```python
from build123d import *

# Parameters (mm, degrees)
SKETCH1_R           = 9
SKETCH1_R_2         = 6
BOSS_EXTRUDE1_DEPTH = 30


with BuildPart() as part:
    # Sketch1 → Boss-Extrude1 (new body)
    # profile 1 of 3: a face of its own
    with BuildSketch(Plane.XY):
        Circle(SKETCH1_R)
        Circle(SKETCH1_R_2, mode=Mode.SUBTRACT)
    # profile 2 of 3: a face of its own
    with BuildSketch(Plane.XY):
        with BuildLine():
            Line((-3.31662479, -5), (-3.31662479, 5))
            ThreePointArc((-3.31662479, 5), (-6, 0), (-3.31662479, -5))
        make_face()
    # profile 3 of 3: a face of its own
    with BuildSketch(Plane.XY):
        with BuildLine():
            ThreePointArc((6, 0), (5.286764074, 2.837274331), (3.31662479, 5))
            Line((3.31662479, 5), (3.31662479, -5))
            ThreePointArc((3.31662479, -5), (5.286764074, -2.837274331), (6, 0))
        make_face()
    extrude(amount=BOSS_EXTRUDE1_DEPTH)


solid = part.part
```
Geometry: final body of the model. Coordinates: model frame, mm. A direction names the side the tool comes from. Round coordinates to 2 decimals unless told otherwise and drop trailing zeros. Loops run counter-clockwise (first coordinate to the right, second up) from the corner with the lowest first, then second, coordinate; pieces in that order, holes last. Notation, with made-up numbers: (39, 44) -> (86, 44) arc R27 ccw to (86, 72) -> close; hole circle Ø4 at (41.5, 58.5). An arc over 180 degrees is marked (long way). Use one line per item in the form item = value.
Item 1: Cut plane B-B on x = 0. Output: boundary loops of the cut face in (y, z).
Evaluation:
outline = (-9, 0) -> (-6, 0) -> (-6, 30) -> (-9, 30) -> close; (6, 0) -> (9, 0) -> (9, 30) -> (6, 30) -> close
Item 2: Cut plane A-A on y = 0. Output: boundary loops of the cut face in (x, z), then the cut area to 3 significant figures.
Evaluation:
outline = (-9, 0) -> (-3.32, 0) -> (-3.32, 30) -> (-9, 30) -> close; (3.32, 0) -> (9, 0) -> (9, 30) -> (3.32, 30) -> close
area = 341 mm2
Item 3: Access query for faces 4 (the flat face through (4, 0, 0)), 5 (the cylindrical face through (0, 6, 15)). Directions: +Z, -Z, +X, -X, +Y, -Y. A direction counts if a zero-diameter tool reaches every point of the face in a straight line with its end or side. Return the directions, or none.
Evaluation:
face_4 = -Z, +X, -X, +Y, -Y
face_5 = +Z, -Z
Item 4: Cut plane C-C on z = 9.75. Output: boundary loops of the cut face in (x, y), then the cut area to 3 significant figures.
Evaluation:
outline = circle Ø18 at (0, 0); hole (-3.32, -5) arc R6 ccw to (3.32, -5) -> (3.32, 5) arc R6 ccw to (-3.32, 5) -> close
area = 179 mm2
Item 5: Material intervals for probe 1 along X at (y, z) = (5.5, 7.25); probe 2 along X at (y, z) = (1.5, 20.5); probe 3 along Y at (x, z) = (2.5, 8.25), sorted ascending.
Evaluation:
probe_1 = -7.12 to -2.4, 2.4 to 7.12
probe_2 = -8.87 to -3.32, 3.32 to 8.87
probe_3 = -8.65 to -5.45, 5.45 to 8.65
Item 6: Cut plane D-D on x = -8. Output: boundary loops of the cut face in (y, z), then the cut area to 3 significant figures.
Evaluation:
outline = (-4.12, 0) -> (4.12, 0) -> (4.12, 30) -> (-4.12, 30) -> close
area = 247 mm2
Item 7: Draft query along Y for faces 1 (the flat face through (3.317, 0, 15)), 2 (the cylindrical face through (-1.172, 8.923, 14.79)), 3 (the flat face through (4, 0, 30)). Return one class per face: released by +Y, released by -Y, zero draft, split by the parting line, or undercut.
Evaluation:
face_1 = undercut
face_2 = split by the parting line
face_3 = zero draft
Item 8: Contact query for flat-ended pins moving along their axis: pin 1 Ø1 at (y, z) = (5.5, 11.5) entering from +X; pin 2 Ø3 at (x, z) = (2, 12) entering from +Y; pin 3 Ø8 at (x, z) = (-5, 4) entering from -Y. Output: stop coordinate, or through.
Evaluation:
pin_1 = 7.48
pin_2 = 8.99
pin_3 = -8.94
